from build123d import *

# Parameters (mm, degrees)
F0_R     = 50.8
F1_DEPTH = 177.8
F4_R     = 12.7
F5_T     = -2.54


with BuildPart() as f1:
    # F0 (on Top) → F1 (new body)
    with BuildSketch(Plane.XY):
        Circle(F0_R)
    extrude(amount=F1_DEPTH)

    # F2 (on Front) → F3 (revolve)
    with BuildSketch(Plane.XZ):
        Polygon((-50.8, 177.8), (0, 177.8), (0, 228.6), (-25.4, 228.6), (-25.4, 199.113131), align=None)
    revolve(axis=Axis((0, 0, 203.2), (0, 0, -1)))

    # F4
    f4_edges = [f1.edges().sort_by_distance(p)[0] for p in [
        (-50.8, 0, 0),
        (0, -50.8, 177.8),
        (0, 50.8, 177.8),
        (25.4, 0, 199.113131),
    ]]
    fillet(f4_edges, radius=F4_R)

    # F5
    f5_openings = [f1.faces().sort_by_distance(p)[0] for p in [
        (0, 0, 228.6),
    ]]
    offset(amount=F5_T, openings=f5_openings)


solid = f1.part
The listing builds one solid part. Answer for the finished solid, in the listing's coordinates (mm). A direction names the side the tool comes from. Give positions to 0.01 mm unless a question says otherwise; leave off trailing zeros. Loops run counter-clockwise (first coordinate to the right, second up) from the corner with the lowest first, then second, coordinate; pieces in that order, holes last. Notation, with made-up numbers: M 35,82 L 81,82 A11 cw 81,92 Z; hole C 61.5,-0.75 d11. An arc over 180 degrees is marked long. Answer as CSV lines item,"result".
Item 1: Which of the six approach directions +Z, -Z, +X, -X, +Y, -Y give full straight-line access (tool end or side, diameter ignored) to faces 1 (the flat face through (-1, 1, 2.54)), 2 (the cylindrical face through (2.976, 22.665, 216.653)), 3 (the cylindrical face through (-11.012, -49.592, 91.175))?
Values follow:
face 1,"none"
face 2,"+Z"
face 3,"+Z, -Z"
Item 2: The part is cut by section A-A (z = 67.5). Give the vertices of the cut face in (x, y), and give its area (3 significant figures).
Values follow:
outline,"C 0,0 d101.6; hole C 0,0 d96.52"
area,"790 mm^2"
Item 3: Given pin 1 Ø8 at (x, z) = (-36.5, 116) entering from +Y; pin 2 Ø12 at (x, y) = (26.5, 11) entering from -Z; pin 3 Ø4 at (y, z) = (-18.5, 197.5) entering from +X; pin 4 Ø6 at (x, y) = (-40, -23.5) entering from -Z, each flat-ended and moving along its own axis, determine where each tip first touches the part or whether it passes through.
Values follow:
pin 1,"stops at y = 39.04"
pin 2,"stops at z = 0"
pin 3,"stops at x = 23.64"
pin 4,"stops at z = 1.16"
Item 4: The mould has two halves that part along Z. Classify faces 4 (the flat face through (-1, 1, 0)), 5 (the conical face through (-29.53, 9.3, 194.45)), 6 (the cylindrical face through (46.03, 14.5, 91.18)): released by +Z, released by -Z, zero draft, split by the parting line, or undercut.
Values follow:
face 4,"released by -Z"
face 5,"released by +Z"
face 6,"undercut"
Item 5: Straight lines are drawn through the part: line 1 along Y through (x, z) = (0, 119); line 2 along Y through (x, z) = (0, 221.25); line 3 along X through (y, z) = (-1.5, 62.5). For each, find the intervals that lie inside material, in ascending order. Write a range as [from, to].
Values follow:
line 1,"y = [-50.8, -48.26], [48.26, 50.8]"
line 2,"y = [-25.4, -22.86], [22.86, 25.4]"
line 3,"x = [-50.78, -48.24], [48.24, 50.78]"
